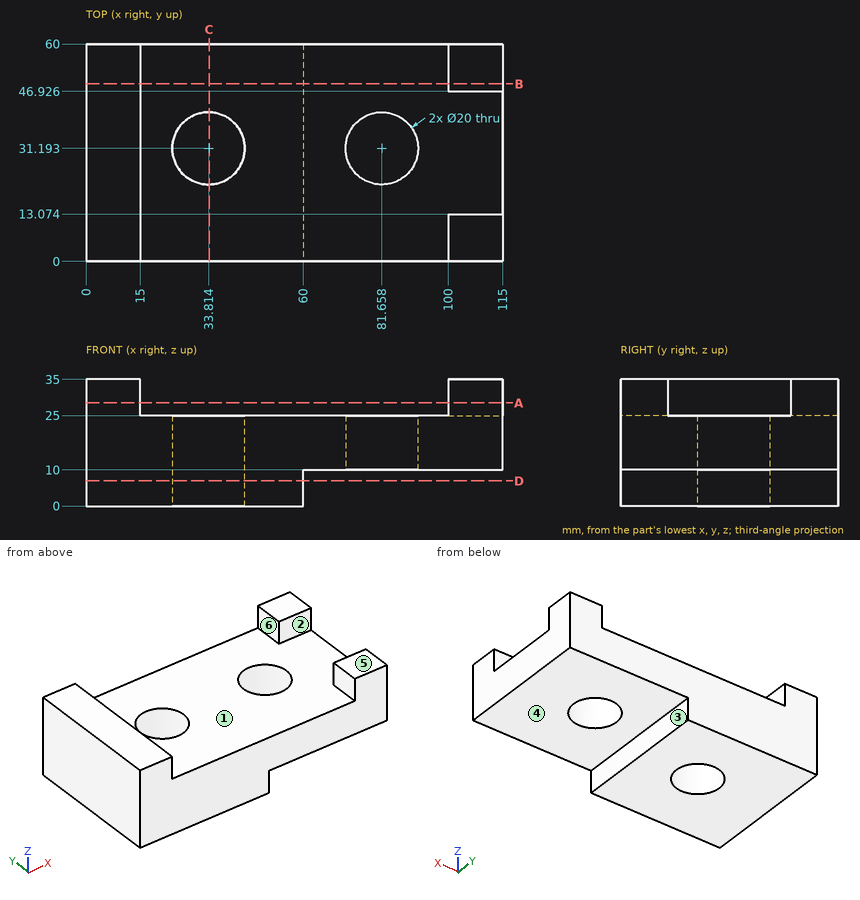
Print and shaded views of the part. All mm, measured from the part's lowest x, y and z. A direction names the side the tool comes from. Give positions to 0.01 mm unless a question says otherwise; leave off trailing zeros. Loops run counter-clockwise (first coordinate to the right, second up) from the corner with the lowest first, then second, coordinate; pieces in that order, holes last.
1) Tool access for the marked faces 4, 5 and 6: list every direction of +Z, -Z, +X, -X, +Y, -Y with a clear straight run to the whole face (end or side of a thin tool).
2) Saw through at A-A (z = 28.5). Write the cut outline in (x, y), plus the area to 3 significant figures.
3) Saw through at D-D (z = 7). Write the cut outline in (x, y), plus the area to 3 significant figures.
4) Saw through at C-C (x = 34). Write the cut outline in (y, z) (1 decimal), plus the area to 3 significant figures.
5) Pull direction X, two halves, no side cores. Call the marked faces 1, 2 and 3: +X half, -X half, draft (parallel to the pull), parting line (faces both ways), or undercut.
6) Saw through at B-B (y = 49). Write the cut outline in (x, z), plus the area to 4 significant figures.
7) Wall check: line 1 (X direction, y = 38, z = 12) (1 decimal); line 2 (X direction, y = 36, z = 20.5) (1 decimal); line 3 (X direction, y = 14, z = 5.5). Give the ranges that are in metal, low to high.
8) Flat gauge pins, fed straight in: pin 1 Ø12 at (x, y) = (81.66, 31.19) entering from +Z; pin 2 Ø3 at (y, z) = (29.5, 3.5) entering from +X; pin 3 Ø8 at (x, y) = (63, 34) entering from +Z. Where does each tip first touch, or does it go through?
Answer block:
1. face 4: -Z, +X, +Y, -Y
1. face 5: +Z, +X, -X, +Y, -Y
1. face 6: +Z, +Y, -Y
2. outline: (0, 0) - (15, 0) - (15, 60) - (0, 60) - close; (100, 0) - (115, 0) - (115, 13.07) - (100, 13.07) - close; (100, 46.93) - (115, 46.93) - (115, 60) - (100, 60) - close
2. area: 1,290 mm2
3. outline: (0, 0) - (60, 0) - (60, 60) - (0, 60) - close; hole circle Ø20 at (33.81, 31.19)
3. area: 3,290 mm2
4. outline: (0, 0) - (21.2, 0) - (21.2, 25) - (0, 25) - close; (41.2, 0) - (60, 0) - (60, 25) - (41.2, 25) - close
4. area: 1,000 mm2
5. face 1: undercut
5. face 2: draft
5. face 3: +X half
6. outline: (0, 0) - (60, 0) - (60, 10) - (115, 10) - (115, 35) - (100, 35) - (100, 25) - (15, 25) - (15, 35) - (0, 35) - close
6. area: 2,625 mm2
7. line 1: x = 0 to 26.5, 41.1 to 74.3, 89 to 115
7. line 2: x = 0 to 25, 42.6 to 72.9, 90.4 to 115
7. line 3: x = 0 to 60
8. pin 1: passes through
8. pin 2: stops at x = 60
8. pin 3: stops at z = 25
